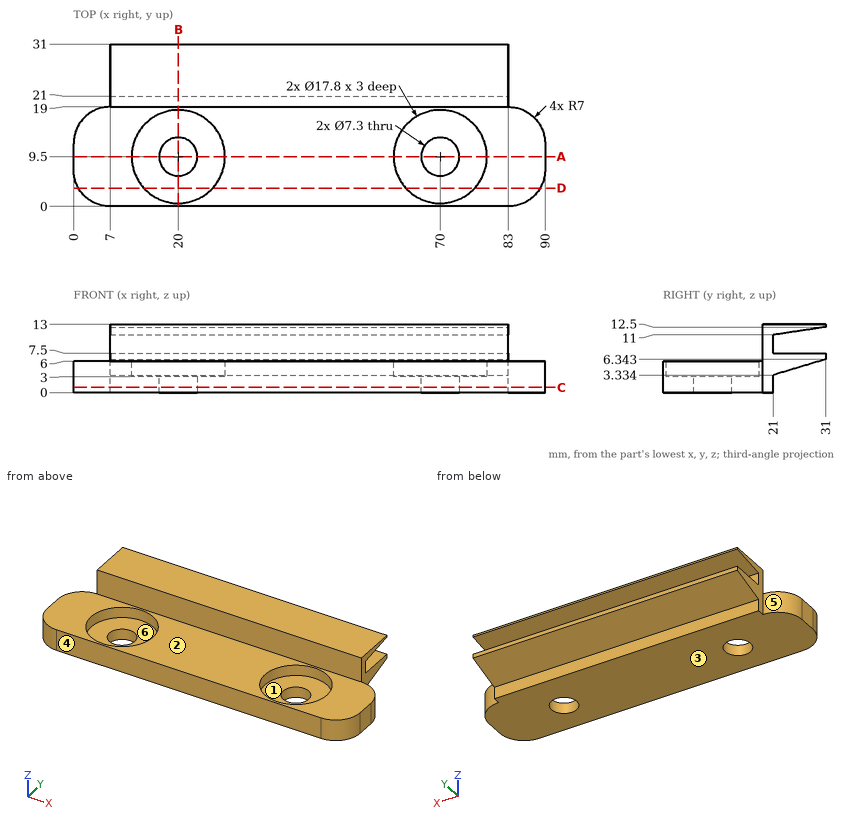
Geometry check sheet. Reference: drawing and pictorial views, mm from the part's lowest x, y, z. A direction names the side the tool comes from. Give positions to 0.01 mm unless a question says otherwise; leave off trailing zeros. Order: outer loops, then holes, each group sorted by start corner. A loop starts at its lowest first (then second) coordinate and runs counter-clockwise, first axis right, second up. Notation, with made-up numbers: M 46.25,38.25 L 92.25,38.25 A17 ccw 92.25,64.25 Z; hole C -38,57 d9. An arc over 180 degrees is marked long. Return JSON: item names as keys, results as strings. Group by question number.
1) Go/stop test with flat-tipped pins: pin 1 Ø7.5 at (x, z) = (63.5, 10.5) entering from -Y; pin 2 Ø3.5 at (y, z) = (28, 8) entering from -X; pin 3 Ø16 at (x, y) = (70, 9.5) entering from +Z. Record where each tip stops, or that it passes through.
2) Section check D-D on y = 3.5. Record the cut outline in (x, z).
3) Mould release check, pull along X, two halves, no side actions. Record for the marked faces 4, 5 and 6: pulls with the +X half, pulls with the -X half, needs draft (parallel to the pull), parting line crosses it, or undercut.
4) Access from +Z, -Z, +X, -X, +Y, -Y to the whole of each face (thin tool, end or side, straight path). Record for the marked faces 1, 2 and 3.
5) Section check A-A on y = 9.5. Record the cut outline in (x, z), and give its area (3 significant figures).
6) Scan lines: line 1 (Y direction, x = 70, z = 1.65); line 2 (X direction, y = 19.5, z = 3.5); line 3 (Z direction, x = 46, y = 1). Record each from-to range of solid material in increasing order.
7) Section check C-C on z = 1. Record the cut outline in (x, y), and give its area (3 significant figures).
8) Section check B-B on x = 20. Record the cut outline in (y, z), and give its area (3 significant figures).
Answer block:
{
 "1": {"pin 1": "stops at y = 19", "pin 2": "stops at x = 7", "pin 3": "stops at z = 3"},
 "2": {"outline": "M 0.94,0 L 89.06,0 L 89.06,6 L 76.57,6 L 76.57,3 L 63.43,3 L 63.43,6 L 26.57,6 L 26.57,3 L 13.43,3 L 13.43,6 L 0.94,6 Z"},
 "3": {"face 4": "needs draft", "face 5": "pulls with the -X half", "face 6": "undercut"},
 "4": {"face 1": "+Z", "face 2": "+Z, +X, -X, -Y", "face 3": "-Z, +X, -X, +Y, -Y"},
 "5": {"outline": "M 0,0 L 16.35,0 L 16.35,3 L 11.1,3 L 11.1,6 L 0,6 Z; M 23.65,0 L 66.35,0 L 66.35,3 L 61.1,3 L 61.1,6 L 28.9,6 L 28.9,3 L 23.65,3 Z; M 73.65,0 L 90,0 L 90,6 L 78.9,6 L 78.9,3 L 73.65,3 Z", "area": "389 mm^2"},
 "6": {"line 1": "y = 0 to 5.85, 13.15 to 21", "line 2": "x = 7 to 83", "line 3": "z = 0 to 6"},
 "7": {"outline": "M 0,7 A7 ccw 7,0 L 83,0 A7 ccw 90,7 L 90,12 A7 ccw 83,19 L 83,21 L 7,21 L 7,19 A7 ccw 0,12 Z; hole C 20,9.5 d7.3; hole C 70,9.5 d7.3", "area": "1,740 mm^2"},
 "8": {"outline": "M 0,0 L 5.85,0 L 5.85,3 L 0.6,3 L 0.6,6 L 0,6 Z; M 13.15,0 L 21,0 L 21,3.33 L 31,6.34 L 31,7.5 L 21,7.5 L 21,11 L 31,12.5 L 31,13 L 19,13 L 19,6 L 18.4,6 L 18.4,3 L 13.15,3 Z", "area": "104 mm^2"}
}
